Here's how the part is built. I have some questions about the finished solid (model axes, mm). Face numbers are marked on the shaded views. A direction names the side the tool comes from. Give positions to 0.01 mm unless a question says otherwise; leave off trailing zeros. Order: outer loops, then holes, each group sorted by start corner. A loop starts at its lowest first (then second) coordinate and runs counter-clockwise, first axis right, second up. Notation, with made-up numbers: (12, 69.25) -> (60, 69.25) arc R17 ccw to (60, 99.25) -> close; hole circle Ø5 at (78.5, 26.25). An arc over 180 degrees is marked (long way). Write each question's results on one line, items separated by ' | '. Start each with the question number.
Q1. Thinking about a two-plate mould opening in Y: for the marked faces 5, 6 and 7, which applies, pulls with the +Y half, pulls with the -Y half, needs draft (parallel to the pull), parting line crosses it, or undercut?
Q2. Imagine slicing it at C-C, the plane z = -45. Please give me the cut outline in (x, y).
Q3. I'm going to push flat-ended pins straight in: pin 1 (9 mm diameter, centred on x = 82, y = -70, fed in from +Z); pin 2 (24 mm diameter, centred on x = -92.5, y = -102.5, fed in from -Z); pin 3 (12 mm diameter, centred on y = -437.5, z = -45, fed in from +X); pin 4 (13.5 mm diameter, centred on x = -75, z = -75, fed in from -Y). Where does each tip first touch, or does it pass through?
Q4. For the marked faces 1, 2, 3 and 4, which set-ups out of +Z, -Z, +X, -X, +Y, -Y let a thin tool reach every point of the face, with its end or its side?
Q5. Imagine slicing it at D-D, the plane y = -340. Please give me the cut outline in (x, z), then the cut area to 3 significant figures.
Q6. I need wall thicknesses on line 1 along Z through (x, y) = (75, -654); line 2 along Y through (x, z) = (-65, 50.5); line 3 along Z through (x, y) = (0, -314). Which ranges of each line are inside material? Lowest first, please. Write a range as [from, to].
Q7. Imagine slicing it at A-A, the plane y = -601. Please give me the cut outline in (x, z).
Q8. Imagine slicing it at B-B, the plane x = 25.5. Please give me the cut outline in (y, z), then the cut area to 3 significant figures.
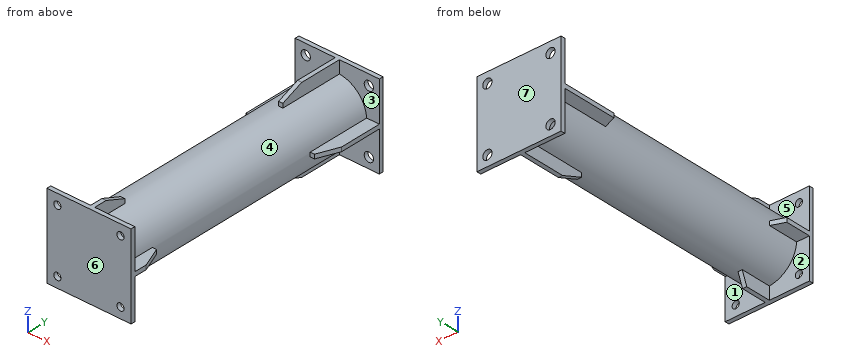
```python
from build123d import *

# Parameters (mm, degrees)
F0_R          = 70
F0_R_2        = 65
F1_DEPTH      = 649
F2_W          = 200
F2_H          = 200
F2_R          = 11
F3_DEPTH      = 10
F4_W          = 30.1787997812
F4_H          = 10
F4_W_2        = 10
F4_H_2        = 30.1787997812
F5_DEPTH      = 150
F6_T1_DEPTH   = 269.311363913
F6_T3_DEPTH   = 269.311363913
F6_T8_DEPTH   = 269.311363913
F6_S9_R       = 70
F6_T10_DEPTH  = 139
F8_W          = 200
F8_H          = 200
F8_R          = 8.5
F9_DEPTH      = 10
F10_W         = 10
F10_H         = 30.1787997812
F10_W_2       = 30.1787997812
F10_H_2       = 10
F11_DEPTH     = 80
F12_T1_DEPTH  = 269.311363913
F12_T3_DEPTH  = 269.311363913
F12_T8_DEPTH  = 269.311363913
F12_S9_R      = 70
F12_T10_DEPTH = 139
F12_T14_DEPTH = 269.311363913
F12_S15_R     = 70
F12_T16_DEPTH = 139


# Not quite as in the source:
# - a fillet or chamfer that OpenCascade refuses, or shapes differently, is made with other operations: its cross-section is extruded or revolved along the edge and cut away or added


with BuildPart() as f1:
    # F0 (on Front) → F1 (new body)
    with BuildSketch(Plane.XZ):
        Circle(F0_R)
        Circle(F0_R_2, mode=Mode.SUBTRACT)
    extrude(amount=F1_DEPTH)

    # F2 (on Front) → F3 (join)
    with BuildSketch(Plane.XZ):
        Rectangle(F2_W, F2_H)
        with Locations((-75, -75)):
            Circle(F2_R, mode=Mode.SUBTRACT)
        with Locations((75, -75)):
            Circle(F2_R, mode=Mode.SUBTRACT)
        with Locations((-75, 75)):
            Circle(F2_R, mode=Mode.SUBTRACT)
        with Locations((75, 75)):
            Circle(F2_R, mode=Mode.SUBTRACT)
    extrude(amount=-F3_DEPTH)

    # F4 (on Front) → F5 (join)
    with BuildSketch(Plane.XZ):
        with Locations((-84.9106001094, 0)):
            Rectangle(F4_W, F4_H)
        with Locations((0, 84.9106001094)):
            Rectangle(F4_W_2, F4_H_2)
        with Locations((84.9106001094, 0)):
            Rectangle(F4_W, F4_H)
        with Locations((0, -84.9106001094)):
            Rectangle(F4_W_2, F4_H_2)
    extrude(amount=F5_DEPTH)

    # F6: chamfer of 50 x 20 on 4 edges, made by hand

    # F6_s2 → F6_t1 (cut)
    with BuildSketch(Plane.YZ.offset(-134.6556819565)):
        Polygon((-100, 100), (-150, 80), (-150, 100), align=None)
        Polygon((-100, -100), (-150, -80), (-150, -100), align=None)
    extrude(amount=F6_T1_DEPTH, mode=Mode.SUBTRACT)

    # F6_s4 → F6_t3 (cut)
    with BuildSketch(Plane.XY.offset(-134.6556819565)):
        Polygon((100, -100), (80, -150), (100, -150), align=None)
    extrude(amount=F6_T3_DEPTH, mode=Mode.SUBTRACT)


with BuildPart() as f6_tool6:
    # F6_s7 → F6_t8 (new body)
    with BuildSketch(Plane.XY.offset(134.6556819565)):
        Polygon((-100, -130), (-50, -150), (-100, -150), align=None)
    extrude(amount=-F6_T8_DEPTH)

    # F6_s9 → F6_t10 (cut, symmetric)
    with BuildSketch(Plane.XZ.offset(140)):
        Circle(F6_S9_R)
    extrude(amount=F6_T10_DEPTH, both=True, mode=Mode.SUBTRACT)


with BuildPart() as f1_1:
    add(f1.part)

    # F6_t5: cut F6_tool6
    add(f6_tool6.part, mode=Mode.SUBTRACT)

    # F8 (on offset) → F9 (join)
    with BuildSketch(Plane.XZ.offset(649)):
        Rectangle(F8_W, F8_H)
        with Locations((-75, -75)):
            Circle(F8_R, mode=Mode.SUBTRACT)
        with Locations((75, -75)):
            Circle(F8_R, mode=Mode.SUBTRACT)
        with Locations((-75, 75)):
            Circle(F8_R, mode=Mode.SUBTRACT)
        with Locations((75, 75)):
            Circle(F8_R, mode=Mode.SUBTRACT)
    extrude(amount=F9_DEPTH)

    # F10 (on face) → F11 (join)
    with BuildSketch(Plane(origin=(0, -649, 0), x_dir=(-1, 0, 0), z_dir=(0, 1, 0))):
        with Locations((0, 84.9106001094)):
            Rectangle(F10_W, F10_H)
        with Locations((84.9106001094, 0)):
            Rectangle(F10_W_2, F10_H_2)
        with Locations((0, -84.9106001094)):
            Rectangle(F10_W, F10_H)
        with Locations((-84.9106001094, 0)):
            Rectangle(F10_W_2, F10_H_2)
    extrude(amount=F11_DEPTH)

    # F12: chamfer of 20 x 50 on 4 edges, made by hand

    # F12_s2 → F12_t1 (cut)
    with BuildSketch(Plane.YZ.offset(-134.6556819565)):
        Polygon((-619, 100), (-569, 80), (-569, 100), align=None)
    extrude(amount=F12_T1_DEPTH, mode=Mode.SUBTRACT)

    # F12_s4 → F12_t3 (cut)
    with BuildSketch(Plane.XY.offset(-134.6556819565)):
        Polygon((100, -619), (80, -569), (100, -569), align=None)
    extrude(amount=F12_T3_DEPTH, mode=Mode.SUBTRACT)


with BuildPart() as f12_tool6:
    # F12_s7 → F12_t8 (new body)
    with BuildSketch(Plane.XY.offset(-134.6556819565)):
        Polygon((-100, -589), (-50, -569), (-100, -569), align=None)
    extrude(amount=F12_T8_DEPTH)

    # F12_s9 → F12_t10 (cut, symmetric)
    with BuildSketch(Plane.XZ.offset(579)):
        Circle(F12_S9_R)
    extrude(amount=F12_T10_DEPTH, both=True, mode=Mode.SUBTRACT)


with BuildPart() as f1_2:
    add(f1_1.part)

    # F12_t5: cut F12_tool6
    add(f12_tool6.part, mode=Mode.SUBTRACT)


with BuildPart() as f12_tool12:
    # F12_s13 → F12_t14 (new body)
    with BuildSketch(Plane.YZ.offset(134.6556819565)):
        Polygon((-589, -100), (-569, -50), (-569, -100), align=None)
    extrude(amount=-F12_T14_DEPTH)

    # F12_s15 → F12_t16 (cut, symmetric)
    with BuildSketch(Plane.XZ.offset(579)):
        Circle(F12_S15_R)
    extrude(amount=F12_T16_DEPTH, both=True, mode=Mode.SUBTRACT)


with BuildPart() as f1_3:
    add(f1_2.part)

    # F12_t11: cut F12_tool12
    add(f12_tool12.part, mode=Mode.SUBTRACT)


solid = f1_3.part
```
Geometry check:
1) face 5: undercut | face 6: pulls with the -Y half | face 7: pulls with the +Y half
2) outline: (-100, -659) -> (100, -659) -> (100, -649) -> (53.62, -649) -> (53.62, 0) -> (100, 0) -> (100, 10) -> (-100, 10) -> (-100, 0) -> (-53.62, 0) -> (-53.62, -649) -> (-100, -649) -> close; hole (-46.9, -649) -> (46.9, -649) -> (46.9, 0) -> (-46.9, 0) -> close
3) pin 1: z = 5 | pin 2: z = -5 | pin 3: x = 58.13 | pin 4: through
4) face 1: -Z, +X | face 2: -Z, -X | face 3: +Z, +X | face 4: none
5) outline: circle Ø140 at (0, 0); hole circle Ø130 at (0, 0) | area: 2,120 mm²
6) line 1: [-100, -83.5], [-66.5, 66.5], [83.5, 100] | line 2: [-659, -649], [0, 10] | line 3: [-70, -65], [65, 70]
7) outline: (-100, -5) -> (-69.82, -5) arc R70 ccw to (-5, -69.82) -> (-5, -100) -> (5, -100) -> (5, -69.82) arc R70 ccw to (69.82, -5) -> (92.8, -5) -> (92.8, 5) -> (69.82, 5) arc R70 ccw to (5, 69.82) -> (5, 92.8) -> (-5, 92.8) -> (-5, 69.82) arc R70 ccw to (-69.82, 5) -> (-100, 5) -> close; hole circle Ø130 at (0, 0)
8) outline: (-659, -100) -> (-649, -100) -> (-649, -65.19) -> (0, -65.19) -> (0, -100) -> (10, -100) -> (10, 100) -> (0, 100) -> (0, 65.19) -> (-649, 65.19) -> (-649, 100) -> (-659, 100) -> close; hole (-649, -59.79) -> (0, -59.79) -> (0, 59.79) -> (-649, 59.79) -> close | area: 11,000 mm²
